Part model, mm, in its own coordinate system. A direction names the side the tool comes from. Give positions to 0.01 mm unless a question says otherwise; leave off trailing zeros. Order: outer loops, then holes, each group sorted by start corner. A loop starts at its lowest first (then second) coordinate and runs counter-clockwise, first axis right, second up. Notation, with made-up numbers: (76, 40.25) - (84, 40.25) arc R18 cw to (84, 47.25) - close; hole circle Ø3 at (-18.5, -27). An arc over 180 degrees is marked (long way). Use a Markdown table: item, result. Add a question column.
from build123d import *

# Parameters (mm, degrees)
BOSS_EXTRUDE3_DEPTH = 320
SKETCH7_W           = 15
SKETCH7_H           = 111
CUT_EXTRUDE3_DEPTH  = 321.702354216
BOSS_EXTRUDE7_DEPTH = 140
SKETCH4_W           = 28
SKETCH4_H           = 78.1
SKETCH4_R           = 3.8
BOSS_EXTRUDE4_DEPTH = 6
BOSS_EXTRUDE8_DEPTH = 10
CUT_EXTRUDE4_DEPTH  = 226.646771605
SKETCH13_R          = 6.8
CUT_EXTRUDE5_DEPTH  = 3


with BuildPart() as part:
    # Sketch1 → Boss-Extrude3 (new body)
    with BuildSketch(Plane(origin=(0, 0, 0), x_dir=(1, 0, 0), z_dir=(0, 1, 0))):
        Polygon((0, 0), (0, 15), (15, 0), align=None)
    extrude(amount=BOSS_EXTRUDE3_DEPTH)

    # Sketch7 → Cut-Extrude3 (cut, through all)
    with BuildSketch(Plane.XY):
        with Locations((7.5, 264.5)):
            Rectangle(SKETCH7_W, SKETCH7_H)
    extrude(amount=-CUT_EXTRUDE3_DEPTH, mode=Mode.SUBTRACT)

    # Sketch10 → Boss-Extrude7 (add)
    with BuildSketch(Plane.XZ):
        Polygon((-3, 3), (-3, -22.242640687), (22.242640687, 3), align=None)
    extrude(amount=-BOSS_EXTRUDE7_DEPTH)

    # Sketch4 → Boss-Extrude4 (add)
    with BuildSketch(Plane.XZ):
        with Locations((11, -36.05)):
            Rectangle(SKETCH4_W, SKETCH4_H)
        with Locations(Location((12.3, -65.04, 0), (0, 0, 270))):
            Circle(SKETCH4_R, mode=Mode.SUBTRACT)
    extrude(amount=-BOSS_EXTRUDE4_DEPTH)

    # Sketch11 → Boss-Extrude8 (add)
    with BuildSketch(Plane(origin=(0, 6, 0), x_dir=(1, 0, 0), z_dir=(0, 1, 0))):
        Polygon((-3, 22.242640687), (4.071067812, 29.313708499), (19.315705646, 14.069070665), (25, 8.384776311), (17.928932188, 1.313708499), align=None)
    extrude(amount=BOSS_EXTRUDE8_DEPTH)

    # Sketch12 → Cut-Extrude4 (cut, through all)
    with BuildSketch(Plane(origin=(8.307611845, 0, 8.307611845), x_dir=(0.7071067811865472, 0, -0.7071067811865479), z_dir=(0.7071067811865479, 0, 0.7071067811865472))):
        with BuildLine():
            Line((13.606601718, 16), (23.606601718, 16))
            Line((23.606601718, 16), (23.606601718, 6))
            ThreePointArc((23.606601718, 6), (16.535533906, 8.928932188), (13.606601718, 16))
        make_face()
    extrude(amount=-CUT_EXTRUDE4_DEPTH, mode=Mode.SUBTRACT)

    # Sketch13 → Cut-Extrude5 (cut)
    with BuildSketch(Plane(origin=(0, 6, 0), x_dir=(1, 0, 0), z_dir=(0, 1, 0))):
        with Locations(Location((12.3, 65.04, 0), (0, 0, 270))):
            Circle(SKETCH13_R)
    extrude(amount=-CUT_EXTRUDE5_DEPTH, mode=Mode.SUBTRACT)


solid = part.part
1. Cut at B-B (y = 142). Write the cut outline in (x, z), plus the area to 4 significant figures.
2. Tool access for faces 5 (the face through (7, 174, -8)), 6 (the face through (0, 174, -7)), 7 (the face through (22, 6, -1)), 8 (the face through (14.343, 4.521, -58.554)), 9 (the face through (8, 174, 0)): list every direction of +Z, -Z, +X, -X, +Y, -Y with a clear straight run to the whole face (end or side of a thin tool).
3. Drill centre lines: probe 1 along X at (y, z) = (1.65, -65.04); probe 2 along Y at (x, z) = (2, -15.5); probe 3 along Y at (x, z) = (14, -42). Where is each one in solid material? Low to high. Write a range as [from, to].
4. Pin check, flat tips, straight feed: P1, Ø7.5, axis at x = 4, y = 174, coming from the +Z side; P2, Ø10, axis at x = 14, z = -26.5, coming from the +Y side; P3, Ø5, axis at x = 14, z = -10.5, coming from the +Y side. Stop position of each tip, or through.
5. Cut at D-D (y = 29). Write the cut outline in (x, z).
6. Mould opens along Z. For faces 1 (the face through (6, 209, -6)), 2 (the face through (11, 3, -75.1)), 3 (the face through (10.84, 1.48, -68.55)), 4 (the face through (8, 69, 3)) say: released by +Z, released by -Z, zero draft, split by the parting line, or undercut.
7. Cut at A-A (z = -65.04). Write the cut outline in (x, y), plus the area to 3 significant figures.
8. Cut at C-C (z = -55.5). Write the cut outline in (x, y), plus the area to 3 significant figures.
Responses:
| question | item | result |
|---|---|---|
| 1 | outline | (0, -15) - (15, 0) - (0, 0) - close |
| 1 | area | 112.5 mm² |
| 2 | face 5 | -Z, +X, +Y |
| 2 | face 6 | +Z, -Z, -X, +Y |
| 2 | face 7 | +X, +Y |
| 2 | face 8 | +Y |
| 2 | face 9 | +Z, +X, -X, +Y |
| 3 | probe 1 | x = [-3, 8.5], [16.1, 25] |
| 3 | probe 2 | y = [0, 140] |
| 3 | probe 3 | y = [0, 6] |
| 4 | P1 | stops at z = 0 |
| 4 | P2 | stops at y = 6 |
| 4 | P3 | stops at y = 11.22 |
| 5 | outline | (-3, -22.24) - (22.24, 3) - (-3, 3) - close |
| 6 | face 1 | zero draft |
| 6 | face 2 | released by -Z |
| 6 | face 3 | undercut |
| 6 | face 4 | released by +Z |
| 7 | outline | (-3, 0) - (8.5, 0) - (8.5, 3) - (5.5, 3) - (5.5, 6) - (-3, 6) - close; (16.1, 0) - (25, 0) - (25, 6) - (19.1, 6) - (19.1, 3) - (16.1, 3) - close |
| 7 | area | 104 mm² |
| 8 | outline | (-3, 0) - (25, 0) - (25, 6) - (-3, 6) - close |
| 8 | area | 168 mm² |
